```python
from build123d import *

# Parameters (mm, degrees)
ESBO_O1_W                = 103
ESBO_O1_H                = 55
RESSALTO_EXTRUS_O1_DEPTH = 3
ESBO_O2_W                = 3
ESBO_O2_H                = 15
CORTE_EXTRUS_O1_DEPTH    = 59.459387612
ESBO_O3_W                = 37
ESBO_O3_H                = 3
CORTE_EXTRUS_O2_DEPTH    = 59.459387612
ESBO_O4_W                = 97
ESBO_O4_H                = 10
CORTE_EXTRUS_O3_DEPTH    = 10


with BuildPart() as part:
    # Esboço1 → Ressalto-extrusão1 (new body)
    with BuildSketch(Plane.XY):
        Rectangle(ESBO_O1_W, ESBO_O1_H)
    extrude(amount=RESSALTO_EXTRUS_O1_DEPTH)

    # Esboço2 → Corte-extrusão1 (cut, through all)
    with BuildSketch(Plane(origin=(0, 0, 0), x_dir=(-1, 0, 0), z_dir=(0, 0, -1))):
        with Locations((-50, 20)):
            Rectangle(ESBO_O2_W, ESBO_O2_H)
        with Locations((-50, -20)):
            Rectangle(ESBO_O2_W, ESBO_O2_H)
        with Locations((50, 20)):
            Rectangle(ESBO_O2_W, ESBO_O2_H)
        with Locations((50, -20)):
            Rectangle(ESBO_O2_W, ESBO_O2_H)
    extrude(amount=-CORTE_EXTRUS_O1_DEPTH, mode=Mode.SUBTRACT)

    # Esboço3 → Corte-extrusão2 (cut, through all)
    with BuildSketch(Plane(origin=(0, 0, 0), x_dir=(-1, 0, 0), z_dir=(0, 0, -1))):
        with Locations((0, -26)):
            Rectangle(ESBO_O3_W, ESBO_O3_H)
    extrude(amount=-CORTE_EXTRUS_O2_DEPTH, mode=Mode.SUBTRACT)

    # Esboço4 → Corte-extrusão3 (cut)
    with BuildSketch(Plane(origin=(0, 0, 0), x_dir=(-1, 0, 0), z_dir=(0, 0, -1))):
        with Locations((0, 22.5)):
            Rectangle(ESBO_O4_W, ESBO_O4_H)
    extrude(amount=-CORTE_EXTRUS_O3_DEPTH, mode=Mode.SUBTRACT)


solid = part.part
```
Part model, mm, in its own coordinate system. A direction names the side the tool comes from. Round coordinates to 2 decimals unless told otherwise and drop trailing zeros. Loops run counter-clockwise (first coordinate to the right, second up) from the corner with the lowest first, then second, coordinate; pieces in that order, holes last. Notation, with made-up numbers: (-4, 85.5) -> (23, 85.5) arc R29 ccw to (23, 107.5) -> close; hole circle Ø5 at (22, 89). An arc over 180 degrees is marked (long way). Use a Markdown table: item, result.
1) Probe line 1 (Y direction, x = -5, z = 2.45); line 2 (X direction, y = 14.5, z = 2.55). List the from-to ranges inside material, lowest first. Write a range as [from, to].
The answers:
| item | result |
|---|---|
| line 1 | y = [-24.5, 17.5] |
| line 2 | x = [-48.5, 48.5] |
2) Cut at B-B, the plane y = -23.5. List the corners of the cut face in (x, z), and give its area (3 significant figures).
The answers:
| item | result |
|---|---|
| outline | (-48.5, 0) -> (48.5, 0) -> (48.5, 3) -> (-48.5, 3) -> close |
| area | 291 mm2 |
3) Cut at A-A, the plane z = 1.25. List the corners of the cut face in (x, y), and give its area (3 significant figures).
The answers:
| item | result |
|---|---|
| outline | (-51.5, -12.5) -> (-48.5, -12.5) -> (-48.5, -27.5) -> (-18.5, -27.5) -> (-18.5, -24.5) -> (18.5, -24.5) -> (18.5, -27.5) -> (48.5, -27.5) -> (48.5, -12.5) -> (51.5, -12.5) -> (51.5, 12.5) -> (48.5, 12.5) -> (48.5, 17.5) -> (-48.5, 17.5) -> (-48.5, 12.5) -> (-51.5, 12.5) -> close |
| area | 4,400 mm2 |
4) Drop flat-ended pins along their axis: pin 1 Ø2 at (x, y) = (29.5, -2) entering from -Z; pin 2 Ø0.9 at (y, z) = (16, 1) entering from +X; pin 3 Ø0.9 at (y, z) = (-21.5, 1.5) entering from -X; pin 4 Ø1.5 at (x, z) = (-6, 2) entering from -Y. Give the stop position or say it passes through.
The answers:
| item | result |
|---|---|
| pin 1 | stops at z = 0 |
| pin 2 | stops at x = 48.5 |
| pin 3 | stops at x = -48.5 |
| pin 4 | stops at y = -24.5 |
5) Pull direction X, two halves, no side cores. Call faces 4 (the flat face through (-1, -5, 3)), 5 (the flat face through (-48.5, 15, 1)), 6 (the flat face through (-18.5, -26, 1)): pulls with the +X half, pulls with the -X half, needs draft (parallel to the pull), parting line crosses it, or undercut.
The answers:
| item | result |
|---|---|
| face 4 | needs draft |
| face 5 | pulls with the -X half |
| face 6 | undercut |
6) Cut at C-C, the plane x = 15. List the corners of the cut face in (y, z), and give its area (3 significant figures).
The answers:
| item | result |
|---|---|
| outline | (-24.5, 0) -> (17.5, 0) -> (17.5, 3) -> (-24.5, 3) -> close |
| area | 126 mm2 |
7) Tool access for faces 1 (the flat face through (48.5, 15, 1)), 2 (the flat face through (48.5, -20, 1)), 3 (the flat face through (-48.5, -20, 1)): list every direction of +Z, -Z, +X, -X, +Y, -Y with a clear straight run to the whole face (end or side of a thin tool).
The answers:
| item | result |
|---|---|
| face 1 | +Z, -Z, +X, +Y |
| face 2 | +Z, -Z, +X, -Y |
| face 3 | +Z, -Z, -X, -Y |
